Geometry: final body of the model. Coordinates: model frame, mm. Give positions to 0.01 mm unless a question says otherwise; leave off trailing zeros. Write each loop counter-clockwise with the first axis right and the second up, starting at its lowest first coordinate (ties: lowest second). Pieces come first, ordered by that corner, then holes. Notation, with made-up numbers: (-29.75, 18.25) - (-3.75, 18.25) arc R13 cw to (-3.75, 25.25) - close; hole circle Ø11 at (81.5, -1). An arc over 180 degrees is marked (long way). Return JSON: item names as keys, results as strings.
from build123d import *

# Parameters (mm, degrees)
BOSS_EXTRUDE1_DEPTH = 0.254
CUT_EXTRUDE1_DEPTH  = 0.254


with BuildPart() as part:
    # Sketch1 → Boss-Extrude1 (new body)
    with BuildSketch(Plane.XY):
        with BuildLine():
            Line((-34.29, 10.033), (31.242, 10.033))
            ThreePointArc((31.242, 10.033), (33.397261469, 9.140261469), (34.29, 6.985))
            Line((34.29, 6.985), (34.29, -6.985))
            ThreePointArc((34.29, -6.985), (33.397261469, -9.140261469), (31.242, -10.033))
            Line((31.242, -10.033), (-34.29, -10.033))
            Line((-34.29, -10.033), (-34.29, 10.033))
        make_face()
    extrude(amount=BOSS_EXTRUDE1_DEPTH)

    # Sketch2 → Cut-Extrude1 (cut)
    with BuildSketch(Plane.XY.offset(0.254)):
        with BuildLine():
            Line((-21.971, 6.223), (21.971, 6.223))
            ThreePointArc((21.971, 6.223), (28.194, 0), (21.971, -6.223))
            Line((21.971, -6.223), (-21.971, -6.223))
            ThreePointArc((-21.971, -6.223), (-28.194, 0), (-21.971, 6.223))
        make_face()
    extrude(amount=-CUT_EXTRUDE1_DEPTH, mode=Mode.SUBTRACT)


solid = part.part
Q1. Material intervals for probe 1 along Y at (x, z) = (9.5, 0.1); probe 2 along X at (y, z) = (2.5, 0.15); probe 3 along X at (y, z) = (-4.75, 0.1), sorted ascending. Write a range as [from, to].
Answer key:
{"probe 1": "y = [-10.03, -6.22], [6.22, 10.03]", "probe 2": "x = [-34.29, -27.67], [27.67, 34.29]", "probe 3": "x = [-34.29, -25.99], [25.99, 34.29]"}
Q2. Section query C-C, the plane z = 0.1. Return the cut outline in (x, y) (3 decimals).
Answer key:
{"outline": "(-34.29, -10.033) - (31.242, -10.033) arc R3.048 ccw to (34.29, -6.985) - (34.29, 6.985) arc R3.048 ccw to (31.242, 10.033) - (-34.29, 10.033) - close; hole (-21.971, -6.223) - (21.971, -6.223) arc R6.223 ccw to (21.971, 6.223) - (-21.971, 6.223) arc R6.223 ccw to start"}
Q3. Section query B-B, the plane y = 4.25. Return the cut outline in (x, z), plus the area to 3 significant figures.
Answer key:
{"outline": "(-34.29, 0) - (-26.52, 0) - (-26.52, 0.25) - (-34.29, 0.25) - close; (26.52, 0) - (34.29, 0) - (34.29, 0.25) - (26.52, 0.25) - close", "area": "3.95 mm^2"}
Q4. Section query A-A, the plane x = 5. Return the cut outline in (y, z).
Answer key:
{"outline": "(-10.03, 0) - (-6.22, 0) - (-6.22, 0.25) - (-10.03, 0.25) - close; (6.22, 0) - (10.03, 0) - (10.03, 0.25) - (6.22, 0.25) - close"}
